Read the model definition and answer for the solid it produces. Units are mm, in the model's axes. A direction names the side the tool comes from. Coordinates: 2 decimals unless noted, no trailing zeros. Loops run counter-clockwise (first coordinate to the right, second up) from the corner with the lowest first, then second, coordinate; pieces in that order, holes last. Notation, with made-up numbers: M 0.25,-37 L 36.25,-37 A13 ccw 36.25,-32 Z; hole C 8.25,38.5 d4. An arc over 180 degrees is marked long. Use one line per item in the form item = value. Start each with the question number.
1. For a pull along Y with two mould halves and no side action, classify faces 4 (the flat face through (-90.48, 121.27, 3.35)), 5 (the flat face through (-52.225, 4, 3)), 6 (the flat face through (-86, 162.4, 3)) as released by +Y, released by -Y, zero draft, split by the parting line, or undercut.
2. The part is cut by section C-C (x = -33). Give the vertices of the cut face in (y, z).
3. The part is cut by section D-D (y = 52). Give the vertices of the cut face in (x, z), plus the area to 3 significant figures.
4. Flat-ended cylindrical pins translate along their axes: pin 1 (1.3 mm diameter, centred on x = -27, z = 2, fed in from +Y); pin 2 (2 mm diameter, centred on y = 38.5, z = 2, fed in from -X); pin 3 (1 mm diameter, centred on y = 188.5, z = 3.5, fed in from +X). Find the tip coordinate at first contact, or state that the pin passes through.
5. The part is cut by section A-A (y = 174.5). Give the vertices of the cut face in (x, z), plus the area to 3 significant figures.
6. A tool of negligible diameter and unlimited length cuts with its end or side. For faces 1 (the flat face through (-60.46, 110.7, 3.45)), 2 (the flat face through (-78, 36, 3)), 3 (the flat face through (-22.225, 4, 3)), from which of +Z, -Z, +X, -X, +Y, -Y can it reach the whole face along a straight path? Write none if from no direction.
7. The part is cut by section B-B (z = 4). Give the number of separate pieces and of enclosed holes in the cut face, plus the area to 3 significant figures.
8. Find the intervals of material crossed by probe 1 along X at (y, z) = (16, 2.5) (3 decimals); probe 2 along Y at (x, z) = (-22, 2); probe 3 along X at (y, z) = (49.5, 6.75), in increasing order. Write a range as [from, to].
from build123d import *

# Parameters (mm, degrees)
BOSS_EXTRUDE1_DEPTH = 6.8
SKETCH2_W           = 2.085
SKETCH2_H           = 5
SKETCH2_W_2         = 3.55
SKETCH2_H_2         = 8.5
SKETCH2_H_3         = 7.5
CUT_EXTRUDE1_DEPTH  = 6.8
CUT_EXTRUDE2_DEPTH  = 6.8
SKETCH4_R           = 1.75
CUT_EXTRUDE3_DEPTH  = 6.8
FILLET1_R           = 1
FILLET2_R           = 0.5


with BuildPart() as part:
    # Sketch1 → Boss-Extrude1 (new body)
    with BuildSketch(Plane.XY):
        with BuildLine():
            Line((-103, 169.798422238), (-103, 190.436528082))
            ThreePointArc((-103, 190.436528082), (-101.582115005, 195.569490389), (-97.730539592, 199.246862648))
            ThreePointArc((-97.730539592, 199.246862648), (-85.697338027, 202.057615588), (-73.881600239, 198.440073256))
            ThreePointArc((-73.881600239, 198.440073256), (-70.90110432, 195.553704599), (-69.348658208, 191.706057135))
            Line((-69.348658208, 191.706057135), (-64.181209637, 162.4))
            ThreePointArc((-64.181209637, 162.4), (-55.56310459, 141.196422986), (-39, 125.4))
            ThreePointArc((-39, 125.4), (-10.413345727, 95.649656796), (0, 55.726706578))
            Line((0, 55.726706578), (0, 0))
            Line((0, 0), (-78, 0))
            Line((-78, 0), (-78, 72.818559508))
            ThreePointArc((-78, 72.818559508), (-80.849795474, 96.521676613), (-89.23675521, 118.873813001))
            Line((-89.23675521, 118.873813001), (-91.76324479, 123.743168745))
            ThreePointArc((-91.76324479, 123.743168745), (-100.150204526, 146.095305133), (-103, 169.798422238))
        make_face()
    extrude(amount=BOSS_EXTRUDE1_DEPTH)

    # Sketch2 → Cut-Extrude1 (cut)
    with BuildSketch(Plane.XY.offset(6.8)):
        with Locations((-51.1825, 11)):
            Rectangle(SKETCH2_W, SKETCH2_H)
        with Locations((-54, 11)):
            Rectangle(SKETCH2_W_2, SKETCH2_H)
        with Locations((-56.8175, 11)):
            Rectangle(SKETCH2_W, SKETCH2_H)
        with Locations((-54, 4.25)):
            Rectangle(SKETCH2_W_2, SKETCH2_H_2)
        with Locations((-54, 17.25)):
            Rectangle(SKETCH2_W_2, SKETCH2_H_3)
        with Locations((-26.8175, 11)):
            Rectangle(SKETCH2_W, SKETCH2_H)
        with Locations((-21.1825, 11)):
            Rectangle(SKETCH2_W, SKETCH2_H)
        with Locations((-24, 17.25)):
            Rectangle(SKETCH2_W_2, SKETCH2_H_3)
        with Locations((-24, 11)):
            Rectangle(SKETCH2_W_2, SKETCH2_H)
        with Locations((-24, 4.25)):
            Rectangle(SKETCH2_W_2, SKETCH2_H_2)
    extrude(amount=-CUT_EXTRUDE1_DEPTH, mode=Mode.SUBTRACT)

    # Sketch3 → Cut-Extrude2 (cut)
    with BuildSketch(Plane.XY.offset(6.8)):
        Polygon((-89.2, 187.4), (-89.2, 189.4), (-82.3, 189.4), (-82.3, 187.4), (-79, 187.4), (-79, 162.4), (-92.5, 162.4), (-92.5, 187.4), align=None)
    extrude(amount=-CUT_EXTRUDE2_DEPTH, mode=Mode.SUBTRACT)

    # Sketch4 → Cut-Extrude3 (cut)
    with BuildSketch(Plane.XY.offset(6.8)):
        with Locations((-74.000212357, 134.060889132)):
            Circle(SKETCH4_R)
        Polygon((-84.488, 145.326270189), (-80.488, 138.398066959), (-74.512424714, 141.848066959), (-78.512424714, 148.776270189), align=None)
        Polygon((-63.488, 108.95320323), (-59.488, 102.025), (-53.512424714, 105.475), (-57.512424714, 112.40320323), align=None)
    extrude(amount=-CUT_EXTRUDE3_DEPTH, mode=Mode.SUBTRACT)

    # Fillet1
    fillet1_edges = [part.edges().sort_by_distance(p)[0] for p in [
        (-79, 162.4, 3.4),
        (-92.5, 162.4, 3.4),
    ]]
    fillet(fillet1_edges, radius=FILLET1_R)

    # Fillet2
    fillet2_edges = [part.edges().sort_by_distance(p)[0] for p in [
        (-50.14, 13.5, 3.4),
        (-50.14, 8.5, 3.4),
        (-57.86, 8.5, 3.4),
        (-57.86, 13.5, 3.4),
        (-55.775, 21, 3.4),
        (-52.225, 21, 3.4),
        (-27.86, 8.5, 3.4),
        (-27.86, 13.5, 3.4),
        (-25.775, 21, 3.4),
        (-22.225, 21, 3.4),
        (-20.14, 13.5, 3.4),
        (-20.14, 8.5, 3.4),
    ]]
    fillet(fillet2_edges, radius=FILLET2_R)


solid = part.part
Computed values:
q1.face_4 = released by -Y
q1.face_5 = zero draft
q1.face_6 = undercut
q2.outline = M 0,0 L 121.34,0 L 121.34,6.8 L 0,6.8 Z
q3.outline = M -78,0 L 0,0 L 0,6.8 L -78,6.8 Z
q3.area = 530 mm²
q4.pin_1 = 117.01
q4.pin_2 = -78
q4.pin_3 = -68.7
q5.outline = M -103,0 L -92.5,0 L -92.5,6.8 L -103,6.8 Z; M -79,0 L -66.31,0 L -66.31,6.8 L -79,6.8 Z
q5.area = 158 mm²
q6.face_1 = +Z, -Z
q6.face_2 = +Z, -Z, -X, -Y
q6.face_3 = +Z, -Z, -Y
q7.separate_pieces = 1
q7.enclosed_holes = 4
q7.area = 11,500 mm²
q8.probe_1 = [-78, -55.775], [-52.225, -25.775], [-22.225, 0]
q8.probe_2 = [0, 8.5], [13.5, 111.52]
q8.probe_3 = [-78, 0]
